The listing builds one solid part. Answer for the finished solid, in the listing's coordinates (mm). A direction names the side the tool comes from. Give positions to 0.01 mm unless a question says otherwise; leave off trailing zeros. Order: outer loops, then holes, each group sorted by start corner. A loop starts at its lowest first (then second) coordinate and runs counter-clockwise, first axis right, second up. Notation, with made-up numbers: (19, -31.75) - (74, -31.75) arc R14 cw to (74, -16.75) - close; hole circle Ø3 at (-8.75, 27). An arc over 180 degrees is marked (long way). Use a Markdown table: item, result. Add a question column.
1) For faces 1 (the face through (-69, -1, 99)), 2 (the face through (72, -1, 125)), 3 (the face through (-65, -1, 2)), 4 (the face through (68, -1, 34)), determine the directions among +Z, -Z, +X, -X, +Y, -Y from which every point of the face is accessible in a straight line to the end or side of a thin tool.
2) Straight lines are drawn through the part: line 1 (Y direction, x = 21.5, z = 151); line 2 (X direction, y = -24, z = 151.5); line 3 (X direction, y = 61.5, z = 9). For each, find the intervals that lie inside material, in ascending order.
3) Find section A-A, the plane x = 8.5. Determine the outline of the cut face in (y, z).
4) Flat-ended cylindrical pins translate along their axes: pin 1 (0.5 mm diameter, centred on y = 21, z = 159.5, fed in from +X); pin 2 (1 mm diameter, centred on y = 0, z = 133.5, fed in from +X); pin 3 (12 mm diameter, centred on y = 46.5, z = 130.5, fed in from -X). Find the tip coordinate at first contact, or state that the pin passes through.
from build123d import *

# Parameters (mm, degrees)
SKETCH1_W           = 150
SKETCH1_H           = 160
SKETCH1_W_2         = 130
SKETCH1_H_2         = 140
BOSS_EXTRUDE1_DEPTH = 5
BOSS_EXTRUDE2_DEPTH = 155
BOSS_EXTRUDE3_DEPTH = 154
SKETCH4_W           = 155
SKETCH4_H           = 3
BOSS_EXTRUDE4_DEPTH = 140
SKETCH5_W           = 155
SKETCH5_H           = 3
BOSS_EXTRUDE5_DEPTH = 140


with BuildPart() as part:
    # Sketch1 → Boss-Extrude1 (new body)
    with BuildSketch(Plane.XY):
        Rectangle(SKETCH1_W, SKETCH1_H)
        Rectangle(SKETCH1_W_2, SKETCH1_H_2, mode=Mode.SUBTRACT)
    extrude(amount=BOSS_EXTRUDE1_DEPTH)

    # Sketch2 → Boss-Extrude2 (add)
    with BuildSketch(Plane.XY.offset(5)):
        Polygon((-75, 80), (-70, 80), (-70, 77), (-72, 77), (-72, 75), (-75, 75), align=None)
        Polygon((72, 75), (75, 75), (75, 80), (70, 80), (70, 77), (72, 77), align=None)
        Polygon((75, -75), (75, -80), (70, -80), (70, -77), (72, -77), (72, -75), align=None)
        Polygon((-70, -80), (-70, -77), (-72, -77), (-72, -75), (-75, -75), (-75, -80), align=None)
    extrude(amount=BOSS_EXTRUDE2_DEPTH)

    # Sketch3 → Boss-Extrude3 (add)
    with BuildSketch(Plane(origin=(0, -77, 0), x_dir=(1, 0, 0), z_dir=(0, 1, 0))):
        Polygon((-71, -160), (-72, -155), (-72, -147), (-71, -142), (-71, -134), (-72, -129), (-72, -121), (-71, -116), (-71, -108), (-72, -103), (-72, -95), (-71, -90), (-71, -82), (-72, -77), (-72, -69), (-71, -64), (-71, -56), (-72, -51), (-72, -43), (-71, -38), (-71, -30), (-72, -25), (-72, -17), (-71, -12), (-71, -5), (-68, -5), (-68, -12.297058541), (-69, -17.297058541), (-69, -24.702941459), (-68, -29.702941459), (-68, -38.297058541), (-69, -43.297058541), (-69, -50.702941459), (-68, -55.702941459), (-68, -64.297058541), (-69, -69.297058541), (-69, -76.702941459), (-68, -81.702941459), (-68, -90.297058541), (-69, -95.297058541), (-69, -102.702941459), (-68, -107.702941459), (-68, -116.297058541), (-69, -121.297058541), (-69, -128.702941459), (-68, -133.702941459), (-68, -142.297058541), (-69, -147.297058541), (-69, -154.702941459), (-68.058257973, -159.411651595), (-68.058257973, -160), align=None)
    boss_extrude3 = extrude(amount=BOSS_EXTRUDE3_DEPTH)

    # Mirror1: Boss-Extrude3 across plane
    add(boss_extrude3.mirror(Plane(origin=(0, 0, 0), x_dir=(0, 0, 1), z_dir=(1, 0, 0))))

    # Sketch4 → Boss-Extrude4 (add)
    with BuildSketch(Plane(origin=(-70, 0, 0), x_dir=(0, 0, -1), z_dir=(1, 0, 0))):
        with Locations((-82.5, 78.5)):
            Rectangle(SKETCH4_W, SKETCH4_H)
    extrude(amount=BOSS_EXTRUDE4_DEPTH)

    # Sketch5 → Boss-Extrude5 (add)
    with BuildSketch(Plane(origin=(-70, 0, 0), x_dir=(0, 0, -1), z_dir=(1, 0, 0))):
        with Locations((-82.5, -78.5)):
            Rectangle(SKETCH5_W, SKETCH5_H)
    extrude(amount=BOSS_EXTRUDE5_DEPTH)


solid = part.part
The answers:
| question | item | result |
|---|---|---|
| 1 | face 1 | none |
| 1 | face 2 | +Z, +X |
| 1 | face 3 | +Z, -Z |
| 1 | face 4 | +Z |
| 2 | line 1 | -80 to -77, 77 to 80 |
| 2 | line 2 | -72 to -69, 69 to 72 |
| 2 | line 3 | -71 to -68, 68 to 71 |
| 3 | outline | (-80, 0) - (-70, 0) - (-70, 5) - (-77, 5) - (-77, 160) - (-80, 160) - close; (70, 0) - (80, 0) - (80, 160) - (77, 160) - (77, 5) - (70, 5) - close |
| 4 | pin 1 | x = 71.15 |
| 4 | pin 2 | x = 71.2 |
| 4 | pin 3 | x = -72 |
